```python
from build123d import *

# Parameters (mm, degrees)
SKETCH1_R           = 50
BOSS_EXTRUDE1_DEPTH = 1.59
SKETCH2_R           = 1.75
CUT_EXTRUDE1_DEPTH  = 1.59
SKETCH3_R           = 1.75
SKETCH3_W           = 11.6
SKETCH3_H           = 22.75
CUT_EXTRUDE2_DEPTH  = 10


with BuildPart() as part:
    # Sketch1 → Boss-Extrude1 (new body)
    with BuildSketch(Plane.XY):
        with Locations(Location((0, 0, 0), (0, 0, 180))):
            Circle(SKETCH1_R)
    extrude(amount=BOSS_EXTRUDE1_DEPTH)

    # Sketch2 → Cut-Extrude1 (cut)
    with BuildSketch(Plane.XY.offset(1.59)):
        with Locations((0, 45)):
            Circle(SKETCH2_R)
        with Locations((45, 0)):
            Circle(SKETCH2_R)
        with Locations((0, -45)):
            Circle(SKETCH2_R)
        with Locations((-45, 0)):
            Circle(SKETCH2_R)
    extrude(amount=-CUT_EXTRUDE1_DEPTH, mode=Mode.SUBTRACT)

    # Sketch3 → Cut-Extrude2 (cut)
    with BuildSketch(Plane.XY.offset(1.59)):
        with Locations((0, 8.5)):
            Circle(SKETCH3_R)
        with Locations((0, -21.25)):
            Circle(SKETCH3_R)
        with Locations((0, -6.375)):
            Rectangle(SKETCH3_W, SKETCH3_H)
    extrude(amount=-CUT_EXTRUDE2_DEPTH, mode=Mode.SUBTRACT)


solid = part.part
```
Verification items for the finished model (mm, model axes). Coordinates: 2 decimals unless noted, no trailing zeros. Loops run counter-clockwise (first coordinate to the right, second up) from the corner with the lowest first, then second, coordinate; pieces in that order, holes last. Notation, with made-up numbers: (82.5, 11.5) -> (135.5, 11.5) arc R27 cw to (135.5, 27.5) -> close; hole circle Ø1 at (-0.75, 28). An arc over 180 degrees is marked (long way). Answer in a Markdown table with one row per item.
1) Scan lines: line 1 along Y through (x, z) = (0, 0.65); line 2 along X through (y, z) = (-5, 1.45); line 3 along Y through (x, z) = (-45, 0.3). Record each from-to range of solid material in increasing order. Write a range as from..to.
The answers:
| item | result |
|---|---|
| line 1 | y = -50..-46.75, -43.25..-23, -19.5..-17.75, 5..6.75, 10.25..43.25, 46.75..50 |
| line 2 | x = -49.75..-5.8, 5.8..49.75 |
| line 3 | y = -21.79..-1.75, 1.75..21.79 |
2) Section check B-B (x = -45). Record the cut outline in (y, z), and give its area (3 significant figures).
The answers:
| item | result |
|---|---|
| outline | (-21.79, 0) -> (-1.75, 0) -> (-1.75, 1.59) -> (-21.79, 1.59) -> close; (1.75, 0) -> (21.79, 0) -> (21.79, 1.59) -> (1.75, 1.59) -> close |
| area | 63.7 mm2 |
3) Section check C-C (z = 0.65). Record the cut outline in (x, y), and give its area (3 significant figures).
The answers:
| item | result |
|---|---|
| outline | circle Ø100 at (0, 0); hole circle Ø3.5 at (-45, 0); hole (-5.8, -17.75) -> (5.8, -17.75) -> (5.8, 5) -> (-5.8, 5) -> close; hole circle Ø3.5 at (0, -45); hole circle Ø3.5 at (0, -21.25); hole circle Ø3.5 at (0, 8.5); hole circle Ø3.5 at (0, 45); hole circle Ø3.5 at (45, 0) |
| area | 7,530 mm2 |
4) Section check A-A (y = 0). Record the cut outline in (x, z).
The answers:
| item | result |
|---|---|
| outline | (-50, 0) -> (-46.75, 0) -> (-46.75, 1.59) -> (-50, 1.59) -> close; (-43.25, 0) -> (-5.8, 0) -> (-5.8, 1.59) -> (-43.25, 1.59) -> close; (5.8, 0) -> (43.25, 0) -> (43.25, 1.59) -> (5.8, 1.59) -> close; (46.75, 0) -> (50, 0) -> (50, 1.59) -> (46.75, 1.59) -> close |
5) Draft check along Y on faces 1 (the face through (0.7, 10.4, 0)), 2 (the face through (-47.69, -15.02, 0.78)), 3 (the face through (46.617, -0.67, 0.806)). Enter one of: released by +Y, released by -Y, zero draft, split by the parting line, or undercut.
The answers:
| item | result |
|---|---|
| face 1 | zero draft |
| face 2 | split by the parting line |
| face 3 | undercut |
6) Depth check by flat-ended pin: P1, Ø4, axis at x = 0, y = -45, coming from the +Z side; P2, Ø0.5, axis at y = -8, z = 1, coming from the -X side; P3, Ø0.5, axis at y = -11.5, z = 1, coming from the +X side. Enter the tip coordinate at first touch or a pass-through.
The answers:
| item | result |
|---|---|
| P1 | stops at z = 1.59 |
| P2 | stops at x = -49.4 |
| P3 | stops at x = 48.72 |
